```python
from build123d import *

# Parameters (mm, degrees)
SKETCH1_R                   = 13.335
BOSS_EXTRUDE1_DEPTH         = 16.66875
F_1_4_CLEARANCE_HOLE1_D     = 6.5278
F_1_4_CLEARANCE_HOLE1_DEPTH = 8.671275816


with BuildPart() as part:
    # Sketch1 → Boss-Extrude1 (new body)
    with BuildSketch(Plane.XY):
        with BuildLine():
            Line((-19.05, -40.64), (19.05, -40.64))
            Line((19.05, -40.64), (16.51, 0))
            ThreePointArc((16.51, 0), (0, 16.51), (-16.51, 0))
            Line((-16.51, 0), (-19.05, -40.64))
        make_face()
        Circle(SKETCH1_R, mode=Mode.SUBTRACT)
        with BuildLine():
            Line((-13.892538769, -8.920620301), (-14.883769384, -24.780310151))
            Line((-14.883769384, -24.780310151), (-8.97384088, -31.968724184))
            Line((-8.97384088, -31.968724184), (8.97384088, -31.968724184))
            Line((8.97384088, -31.968724184), (14.883769384, -24.780310151))
            Line((14.883769384, -24.780310151), (13.892538769, -8.920620301))
            ThreePointArc((13.892538769, -8.920620301), (0, -16.51), (-13.892538769, -8.920620301))
        make_face(mode=Mode.SUBTRACT)
    extrude(amount=BOSS_EXTRUDE1_DEPTH)

    # 1/4 Clearance Hole1
    with Locations(Plane(origin=(0, -40.64, 0), x_dir=(-1, 0, 0), z_dir=(0, -1, 0))):
        with Locations((0, -8.334375)):
            Hole(F_1_4_CLEARANCE_HOLE1_D / 2, depth=F_1_4_CLEARANCE_HOLE1_DEPTH)


solid = part.part
```
Input: part model. Units: mm. Frame: model coordinates. A direction names the side the tool comes from. Round coordinates to 2 decimals unless told otherwise and drop trailing zeros. Loops run counter-clockwise (first coordinate to the right, second up) from the corner with the lowest first, then second, coordinate; pieces in that order, holes last.
1) Pin query (flat end, axial travel): pin 1 (2 mm diameter, centred on y = 0, z = 13.5, fed in from +X); pin 2 (2 mm diameter, centred on y = -2.5, z = 9, fed in from +X); pin 3 (5 mm diameter, centred on y = -5, z = 10, fed in from +X). Return the tip coordinate at first contact, or that it passes through.
Ans:
pin 1: stops at x = 16.57
pin 2: stops at x = 16.73
pin 3: stops at x = 16.98
2) Section query D-D on z = 2.5. Return the cut outline in (x, y) (3 decimals).
Ans:
outline: (-19.05, -40.64) - (19.05, -40.64) - (16.51, 0) arc R16.51 ccw to (-16.51, 0) - close; hole (-14.884, -24.78) - (-8.974, -31.969) - (8.974, -31.969) - (14.884, -24.78) - (13.893, -8.921) arc R16.51 cw to (-13.893, -8.921) - close; hole circle Ø26.67 at (0, 0)
3) Material intervals for line 1 (Z direction, x = 0, y = -39); line 2 (X direction, y = 0.5, z = 8.75); line 3 (Y direction, x = -9.5, z = 1.75), sorted ascending.
Ans:
line 1: z = 0 to 5.07, 11.6 to 16.67
line 2: x = -16.5 to -13.33, 13.33 to 16.5
line 3: y = -40.64 to -31.33, -13.5 to -9.36, 9.36 to 13.5
4) Section query C-C on y = -23. Return the cut outline in (x, z).
Ans:
outline: (-17.95, 0) - (-14.77, 0) - (-14.77, 16.67) - (-17.95, 16.67) - close; (14.77, 0) - (17.95, 0) - (17.95, 16.67) - (14.77, 16.67) - close
5) Pull-direction query (X, two-part tool) for faces 4 (the flat face through (8, -12, 16.669)), 5 (the flat face through (-11.97, -28.324, 8.218)), 6 (the flat face through (17.798, -20.604, 8.218)), 7 (the flat face through (-14.38, -16.74, 8.22)); classes: released by +X, released by -X, zero draft, split by the parting line, or undercut.
Ans:
face 4: zero draft
face 5: undercut
face 6: released by +X
face 7: undercut
6) Set-up query: faces 1 (the flat face through (11.89, -28.42, 8.22)), 2 (the flat face through (8, -12, 0)), 3 (the cylindrical face through (-0.71, -36.24, 11.52)). Return all of +Z, -Z, +X, -X, +Y, -Y with unobstructed straight access to the full face (end or side cutting, diameter ignored); none if empty.
Ans:
face 1: +Z, -Z
face 2: -Z, +X, -X, +Y, -Y
face 3: -Y
7) Section query B-B on z = 9.25. Return the cut outline in (x, y) (3 decimals).
Ans:
outline: (-19.05, -40.64) - (-3.133, -40.64) - (-3.133, -31.969) - (-8.974, -31.969) - (-14.884, -24.78) - (-13.893, -8.921) arc R16.51 ccw to (13.893, -8.921) - (14.884, -24.78) - (8.974, -31.969) - (3.133, -31.969) - (3.133, -40.64) - (19.05, -40.64) - (16.51, 0) arc R16.51 ccw to (-16.51, 0) - close; hole circle Ø26.67 at (0, 0)
8) Section query A-A on x = 0. Return the cut outline in (y, z) (3 decimals).
Ans:
outline: (-40.64, 0) - (-31.969, 0) - (-31.969, 5.07) - (-40.64, 5.07) - close; (-40.64, 11.598) - (-31.969, 11.598) - (-31.969, 16.669) - (-40.64, 16.669) - close; (-16.51, 0) - (-13.335, 0) - (-13.335, 16.669) - (-16.51, 16.669) - close; (13.335, 0) - (16.51, 0) - (16.51, 16.669) - (13.335, 16.669) - close
